Source: three-view drawing plus pictorial views. Frame: mm from the lowest corner of the part. Coordinates: 2 decimals unless noted, no trailing zeros. Write each loop counter-clockwise with the first axis right and the second up, starting at its lowest first coordinate (ties: lowest second). Pieces come first, ordered by that corner, then holes. Notation, with made-up numbers: (-14, 18.25) -> (41, 18.25) arc R32 cw to (41, 54.25) -> close; hole circle Ø1 at (20, 40.5). An arc over 180 degrees is marked (long way). One line per item, written item: value.
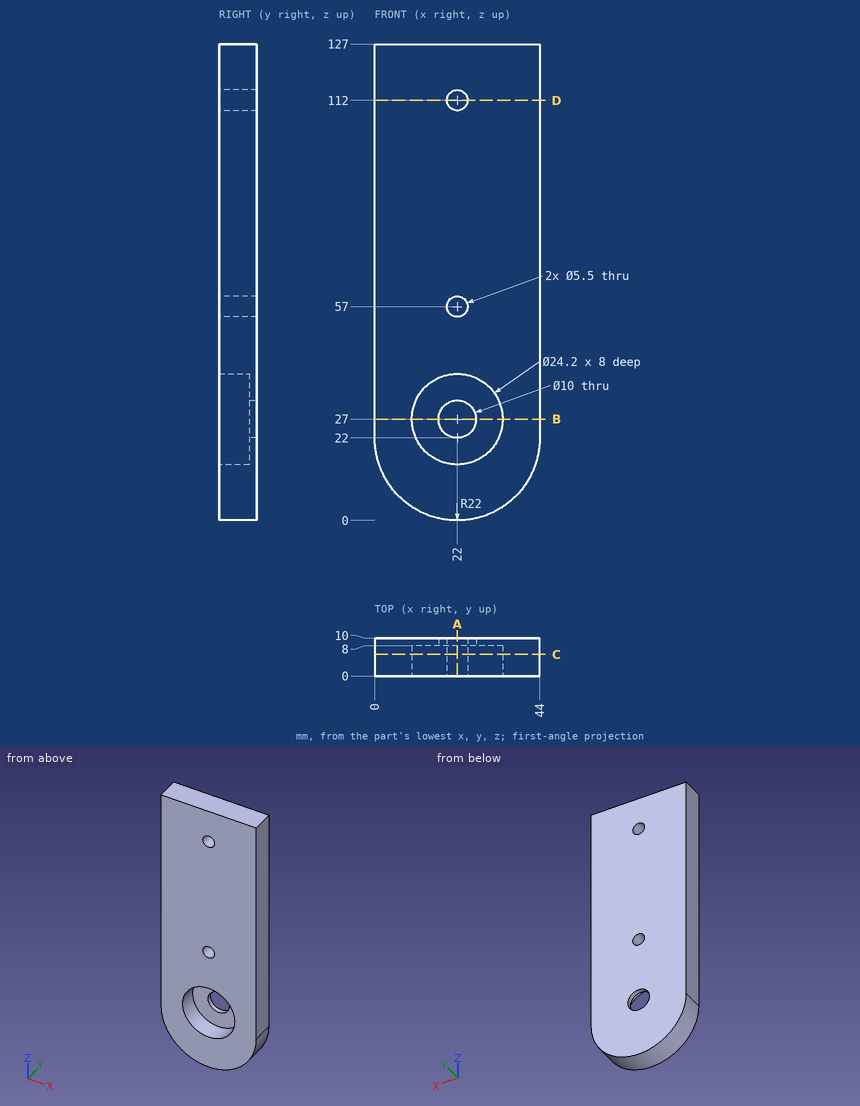
(1) Line query: line 1 (X direction, y = 4, z = 27); line 2 (X direction, y = 3, z = 112); line 3 (Y direction, x = 26, z = 20). Output: solid intervals per line, ascending. Write a range as [from, to].
Responses:
line 1: x = [0, 9.9], [34.1, 44]
line 2: x = [0, 19.25], [24.75, 44]
line 3: y = [8, 10]
(2) Section C-C (y = 5.75). Return the cut outline in (x, z), then the cut area to 3 significant figures.
Responses:
outline: (0, 22) arc R22 ccw to (44, 22) -> (44, 127) -> (0, 127) -> close; hole circle Ø24.2 at (22, 27); hole circle Ø5.5 at (22, 57); hole circle Ø5.5 at (22, 112)
area: 4,870 mm2
(3) Section A-A (x = 22). Return the cut outline in (y, z).
Responses:
outline: (0, 0) -> (10, 0) -> (10, 22) -> (8, 22) -> (8, 14.9) -> (0, 14.9) -> close; (0, 39.1) -> (8, 39.1) -> (8, 32) -> (10, 32) -> (10, 54.25) -> (0, 54.25) -> close; (0, 59.75) -> (10, 59.75) -> (10, 109.25) -> (0, 109.25) -> close; (0, 114.75) -> (10, 114.75) -> (10, 127) -> (0, 127) -> close
(4) Section B-B (z = 27). Return the cut outline in (x, y).
Responses:
outline: (0, 0) -> (9.9, 0) -> (9.9, 8) -> (17, 8) -> (17, 10) -> (0, 10) -> close; (27, 8) -> (34.1, 8) -> (34.1, 0) -> (44, 0) -> (44, 10) -> (27, 10) -> close
(5) Section D-D (z = 112). Return the cut outline in (x, y).
Responses:
outline: (0, 0) -> (19.25, 0) -> (19.25, 10) -> (0, 10) -> close; (24.75, 0) -> (44, 0) -> (44, 10) -> (24.75, 10) -> close
(6) First-contact query: pin 1 (7.5 mm diameter, centred on x = 17, z = 22, fed in from -Y); pin 2 (4.5 mm diameter, centred on x = 22, z = 112, fed in from -Y); pin 3 (1 mm diameter, centred on x = 18.5, y = 6, fed in from -Z). Flat tips, straight axial feed; report the tip coordinate or a pass-through.
Responses:
pin 1: stops at y = 8
pin 2: passes through
pin 3: stops at z = 0.21
